Part print with two shaded views. Sizes in mm from the minimum x, y, z corner. A direction names the side the tool comes from. Coordinates: 2 decimals unless noted, no trailing zeros. Loops run counter-clockwise (first coordinate to the right, second up) from the corner with the lowest first, then second, coordinate; pieces in that order, holes last.
(1) Tool access for the marked faces 1 and 2: list every direction of +Z, -Z, +X, -X, +Y, -Y with a clear straight run to the whole face (end or side of a thin tool).
(2) Slice it at B-B (z = 13.5). Give the cut face in (x, y).
(3) Slice it at C-C (x = 6). Give the cut face in (y, z), and give its area (3 significant figures).
(4) Wall check: L1, parallel to Y at x = 6, z = 49; L2, parallel to Y at x = 3.5, z = 24.5; L3, parallel to X at y = 3.5, z = 69. Give the ranges that are in metal, low to high.
(5) Flat gauge pins, fed straight in: P1, Ø6, axis at y = 22, z = 56.5, coming from the -X side; P2, Ø1.5, axis at y = 2.5, z = 21, coming from the +X side. Where does each tip first touch, or does it go through?
(6) Slice it at A-A (y = 9). Give the cut face in (x, z), and give its area (3 significant figures).
(7) Slice it at D-D (x = 9). Give the cut face in (y, z).
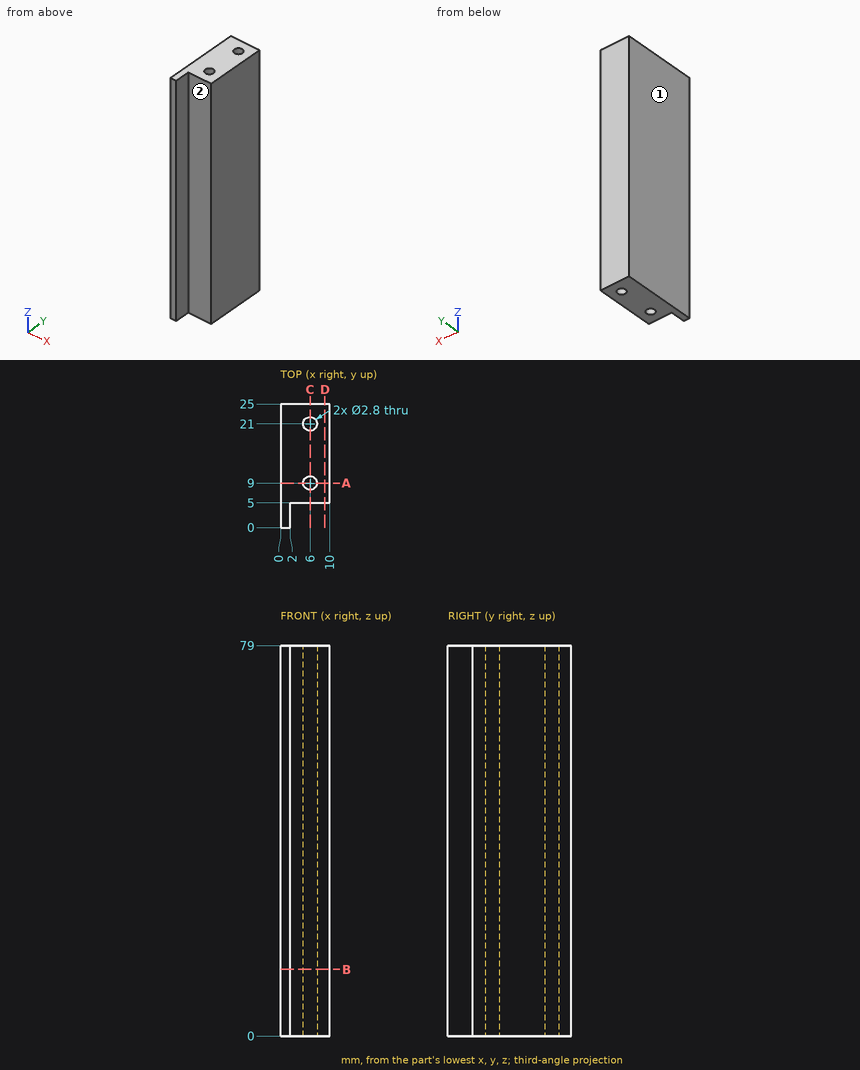
Response values:
1. face 1: +Z, -Z, -X, +Y, -Y
1. face 2: +Z, -Z, +X, -Y
2. outline: (0, 0) - (2, 0) - (2, 5) - (10, 5) - (10, 25) - (0, 25) - close; hole circle Ø2.8 at (6, 9); hole circle Ø2.8 at (6, 21)
3. outline: (5, 0) - (7.6, 0) - (7.6, 79) - (5, 79) - close; (10.4, 0) - (19.6, 0) - (19.6, 79) - (10.4, 79) - close; (22.4, 0) - (25, 0) - (25, 79) - (22.4, 79) - close
3. area: 1,140 mm2
4. L1: y = 5 to 7.6, 10.4 to 19.6, 22.4 to 25
4. L2: y = 5 to 25
4. L3: x = 0 to 2
5. P1: stops at x = 0
5. P2: stops at x = 2
6. outline: (0, 0) - (4.6, 0) - (4.6, 79) - (0, 79) - close; (7.4, 0) - (10, 0) - (10, 79) - (7.4, 79) - close
6. area: 569 mm2
7. outline: (5, 0) - (25, 0) - (25, 79) - (5, 79) - close
